Study the drawing (mm; zero at the part's minimum x, y, z) and answer. A direction names the side the tool comes from. Coordinates: 2 decimals unless noted, no trailing zeros. Loops run counter-clockwise (first coordinate to the right, second up) from the corner with the lowest first, then second, coordinate; pieces in that order, holes last. Notation, with made-up numbers: (-2, 64) - (52, 64) arc R9 ccw to (52, 70) - close; hole circle Ø5 at (-25, 35). An arc over 180 degrees is marked (long way). Use one line per item in the form item = value.
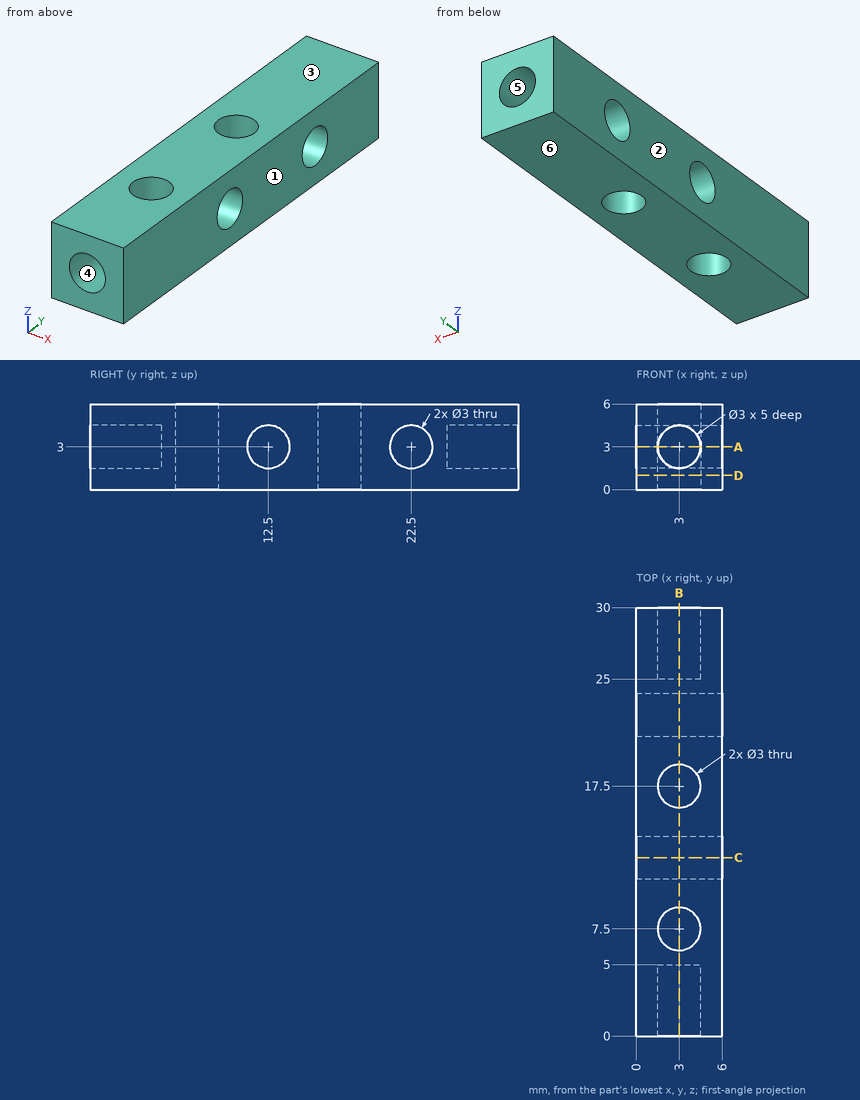
Item 1: The part is cut by section C-C on y = 12.5. Give the vertices of the cut face in (x, z), plus the area to 3 significant figures.
Results below:
outline = (0, 0) - (6, 0) - (6, 1.5) - (0, 1.5) - close; (0, 4.5) - (6, 4.5) - (6, 6) - (0, 6) - close
area = 18.0 mm²
Item 2: The part is cut by section D-D on z = 1. Give the vertices of the cut face in (x, y), plus the area to 3 significant figures.
Results below:
outline = (0, 0) - (6, 0) - (6, 30) - (0, 30) - close; hole circle Ø3 at (3, 7.5); hole circle Ø3 at (3, 17.5)
area = 166 mm²
Item 3: Each of these flat-tipped pins is pushed along its axis until it touches: P1, Ø2.5, axis at x = 3, z = 3, coming from the -Y side; P2, Ø0.9, axis at x = 3.5, z = 3, coming from the +Y side. Where does it stop, or does it pass through?
Results below:
P1 = 5
P2 = 25
Item 4: The part is cut by section B-B on x = 3. Give the vertices of the cut face in (y, z).
Results below:
outline = (0, 0) - (6, 0) - (6, 6) - (0, 6) - (0, 4.5) - (5, 4.5) - (5, 1.5) - (0, 1.5) - close; (9, 0) - (16, 0) - (16, 6) - (9, 6) - close; (19, 0) - (30, 0) - (30, 1.5) - (25, 1.5) - (25, 4.5) - (30, 4.5) - (30, 6) - (19, 6) - close; hole circle Ø3 at (12.5, 3); hole circle Ø3 at (22.5, 3)
Item 5: The part is cut by section A-A on z = 3. Give the vertices of the cut face in (x, y), plus the area to 3 significant figures.
Results below:
outline = (0, 0) - (1.5, 0) - (1.5, 5) - (4.5, 5) - (4.5, 0) - (6, 0) - (6, 11) - (0, 11) - close; (0, 14) - (6, 14) - (6, 21) - (0, 21) - close; (0, 24) - (6, 24) - (6, 30) - (4.5, 30) - (4.5, 25) - (1.5, 25) - (1.5, 30) - (0, 30) - close; hole circle Ø3 at (3, 7.5); hole circle Ø3 at (3, 17.5)
area = 99.9 mm²
Item 6: Find the intervals of material crossed by L1, parallel to Y at x = 4.7, z = 3; L2, parallel to X at y = 2.4, z = 3; L3, parallel to Y at x = 2.4, z = 2.7, in increasing order.
Results below:
L1 = 0 to 11, 14 to 21, 24 to 30
L2 = 0 to 1.5, 4.5 to 6
L3 = 5 to 6.13, 8.87 to 11.03, 13.97 to 16.13, 18.87 to 21.03, 23.97 to 25
Item 7: For a pull along X with two mould halves and no side action, classify the marked faces 1, 2, 3 and 4 as +X half, -X half, draft (parallel to the pull), parting line (faces both ways), or undercut.
Results below:
face_1 = +X half
face_2 = -X half
face_3 = draft
face_4 = undercut
Item 8: Which of the six approach directions +Z, -Z, +X, -X, +Y, -Y give full straight-line access (tool end or side, diameter ignored) to the marked faces 5 and 6?
Results below:
face_5 = +Y
face_6 = -Z, +X, -X, +Y, -Y
